from build123d import *

# Parameters (mm, degrees)
SKETCH1_W           = 152.4
SKETCH1_H           = 101.6
BOSS_EXTRUDE1_DEPTH = 6.35
SKETCH2_R           = 3.81
BOSS_EXTRUDE2_DEPTH = 50.8
SKETCH3_R           = 1.1303
CUT_EXTRUDE2_DEPTH  = 12.7
CUT_EXTRUDE3_DEPTH  = 6.35
SKETCH6_W           = 30.413113892
SKETCH6_H           = 50.8
BOSS_EXTRUDE3_DEPTH = 25.4
SKETCH8_W           = 30.413113892
SKETCH8_H           = 50.8
CUT_EXTRUDE4_DEPTH  = 25.4
SKETCH9_R           = 3.175
CUT_EXTRUDE5_DEPTH  = 2.54
SKETCH10_W          = 19.812
SKETCH10_H          = 64.262
CUT_EXTRUDE6_DEPTH  = 2.54
SKETCH12_R          = 1.1303
CUT_EXTRUDE7_DEPTH  = 132.950059198
FILLET1_R           = 2.54


with BuildPart() as part:
    # Sketch1 → Boss-Extrude1 (new body)
    with BuildSketch(Plane(origin=(0, 0, 0), x_dir=(1, 0, 0), z_dir=(0, 1, 0))):
        with Locations((28.027586207, -12.182445141)):
            Rectangle(SKETCH1_W, SKETCH1_H)
    extrude(amount=BOSS_EXTRUDE1_DEPTH)

    # Sketch2 → Boss-Extrude2 (add)
    with BuildSketch(Plane(origin=(0, 6.35, 0), x_dir=(1, 0, 0), z_dir=(0, 1, 0))):
        with Locations(Location((-44.362413793, 13.217554859, 0), (0, 0, 180))):
            Circle(SKETCH2_R)
        with Locations(Location((-43.092413793, -24.882445141, 0), (0, 0, 270))):
            Circle(SKETCH2_R)
        with Locations(Location((94.067586207, 19.567554859, 0), (0, 0, 270))):
            Circle(SKETCH2_R)
        with Locations(Location((94.067586207, -43.932445141, 0), (0, 0, 270))):
            Circle(SKETCH2_R)
    extrude(amount=BOSS_EXTRUDE2_DEPTH)

    # Sketch3 → Cut-Extrude2 (cut)
    with BuildSketch(Plane(origin=(0, 57.15, 0), x_dir=(1, 0, 0), z_dir=(0, 1, 0))):
        with Locations(Location((-44.362413793, 13.217554859, 0), (0, 0, 270))):
            Circle(SKETCH3_R)
        with Locations(Location((94.067586207, -43.932445141, 0), (0, 0, 270))):
            Circle(SKETCH3_R)
        with Locations(Location((94.067586207, 19.567554859, 0), (0, 0, 270))):
            Circle(SKETCH3_R)
        with Locations(Location((-43.092413793, -24.882445141, 0), (0, 0, 270))):
            Circle(SKETCH3_R)
    extrude(amount=-CUT_EXTRUDE2_DEPTH, mode=Mode.SUBTRACT)

    # Sketch4 → Cut-Extrude3 (cut)
    with BuildSketch(Plane.XZ):
        with BuildLine():
            ThreePointArc((38.123586207, 42.789445141), (37.537799769, 44.203658703), (36.123586207, 44.789445141))
            Line((36.123586207, 44.789445141), (36.123586207, 42.789445141))
            Line((36.123586207, 42.789445141), (36.123586207, 40.789445141))
            ThreePointArc((36.123586207, 40.789445141), (37.537799769, 41.375231579), (38.123586207, 42.789445141))
        make_face()
        with BuildLine():
            Line((36.123586207, 42.789445141), (36.123586207, 44.789445141))
            ThreePointArc((36.123586207, 44.789445141), (34.123586207, 42.789445141), (36.123586207, 40.789445141))
            Line((36.123586207, 40.789445141), (36.123586207, 42.789445141))
        make_face()
        with BuildLine():
            ThreePointArc((38.123586207, 42.789445141), (37.537799769, 44.203658703), (36.123586207, 44.789445141))
            Line((36.123586207, 44.789445141), (36.123586207, 42.789445141))
            Line((36.123586207, 42.789445141), (36.123586207, 40.789445141))
            ThreePointArc((36.123586207, 40.789445141), (37.537799769, 41.375231579), (38.123586207, 42.789445141))
        make_face()
        with BuildLine():
            Line((36.123586207, 42.789445141), (36.123586207, 44.789445141))
            ThreePointArc((36.123586207, 44.789445141), (34.123586207, 42.789445141), (36.123586207, 40.789445141))
            Line((36.123586207, 40.789445141), (36.123586207, 42.789445141))
        make_face()
        with BuildLine():
            ThreePointArc((45.426586207, 42.789445141), (44.840799769, 44.203658703), (43.426586207, 44.789445141))
            Line((43.426586207, 44.789445141), (43.426586207, 42.789445141))
            Line((43.426586207, 42.789445141), (43.426586207, 40.789445141))
            ThreePointArc((43.426586207, 40.789445141), (44.840799769, 41.375231579), (45.426586207, 42.789445141))
        make_face()
        with BuildLine():
            Line((43.426586207, 42.789445141), (43.426586207, 44.789445141))
            ThreePointArc((43.426586207, 44.789445141), (41.426586207, 42.789445141), (43.426586207, 40.789445141))
            Line((43.426586207, 40.789445141), (43.426586207, 42.789445141))
        make_face()
        with BuildLine():
            ThreePointArc((45.426586207, 42.789445141), (44.840799769, 44.203658703), (43.426586207, 44.789445141))
            Line((43.426586207, 44.789445141), (43.426586207, 42.789445141))
            Line((43.426586207, 42.789445141), (43.426586207, 40.789445141))
            ThreePointArc((43.426586207, 40.789445141), (44.840799769, 41.375231579), (45.426586207, 42.789445141))
        make_face()
        with BuildLine():
            Line((43.426586207, 42.789445141), (43.426586207, 44.789445141))
            ThreePointArc((43.426586207, 44.789445141), (41.426586207, 42.789445141), (43.426586207, 40.789445141))
            Line((43.426586207, 40.789445141), (43.426586207, 42.789445141))
        make_face()
    cut_extrude3 = extrude(amount=-CUT_EXTRUDE3_DEPTH, mode=Mode.SUBTRACT)

    # Sketch6 → Boss-Extrude3 (add)
    with BuildSketch(Plane(origin=(0, 6.35, 0), x_dir=(1, 0, 0), z_dir=(0, 1, 0))):
        with Locations((33.36893454, 13.217554859)):
            Rectangle(SKETCH6_W, SKETCH6_H)
    extrude(amount=BOSS_EXTRUDE3_DEPTH)

    # Mirror1: Cut-Extrude3 across plane
    add(cut_extrude3.mirror(Plane(origin=(48.575491486, 31.75, 12.182445141), x_dir=(1, 0, 0), z_dir=(0, 0, -1))), mode=Mode.SUBTRACT)

    # Sketch8 → Cut-Extrude4 (cut)
    with BuildSketch(Plane(origin=(0, 31.75, 0), x_dir=(1, 0, 0), z_dir=(0, 1, 0))):
        with Locations((33.36893454, 13.217554859)):
            Rectangle(SKETCH8_W, SKETCH8_H)
    extrude(amount=-CUT_EXTRUDE4_DEPTH, mode=Mode.SUBTRACT)

    # Sketch9 → Cut-Extrude5 (cut)
    with BuildSketch(Plane(origin=(0, 6.35, 0), x_dir=(1, 0, 0), z_dir=(0, 1, 0))):
        with Locations(Location((43.426586207, 18.424554859, 0), (0, 0, 270))):
            Circle(SKETCH9_R)
        with Locations(Location((36.123586207, 18.424554859, 0), (0, 0, 270))):
            Circle(SKETCH9_R)
        with Locations(Location((43.426586207, -42.789445141, 0), (0, 0, 270))):
            Circle(SKETCH9_R)
        with Locations(Location((36.123586207, -42.789445141, 0), (0, 0, 270))):
            Circle(SKETCH9_R)
    extrude(amount=-CUT_EXTRUDE5_DEPTH, mode=Mode.SUBTRACT)

    # Sketch10 → Cut-Extrude6 (cut)
    with BuildSketch(Plane(origin=(0, 6.35, 0), x_dir=(1, 0, 0), z_dir=(0, 1, 0))):
        with Locations((77.811586207, -9.756234071)):
            Rectangle(SKETCH10_W, SKETCH10_H)
    extrude(amount=-CUT_EXTRUDE6_DEPTH, mode=Mode.SUBTRACT)

    # Sketch12 → Cut-Extrude7 (cut, through all)
    with BuildSketch(Plane(origin=(0, 6.35, 0), x_dir=(1, 0, 0), z_dir=(0, 1, 0))):
        with Locations(Location((-31.662413793, 13.217554859, 0), (0, 0, 270))):
            Circle(SKETCH12_R)
        with Locations(Location((16.597586207, 11.947554859, 0), (0, 0, 270))):
            Circle(SKETCH12_R)
        with Locations(Location((1.357586207, -38.852445141, 0), (0, 0, 270))):
            Circle(SKETCH12_R)
        with Locations(Location((-26.582413793, -38.852445141, 0), (0, 0, 270))):
            Circle(SKETCH12_R)
    extrude(amount=-CUT_EXTRUDE7_DEPTH, mode=Mode.SUBTRACT)

    # Fillet1
    fillet1_edges = [part.edges().sort_by_distance(p)[0] for p in [
        (-48.172413793, 3.175, -38.617554859),
        (104.227586207, 3.175, -38.617554859),
        (104.227586207, 3.175, 62.982445141),
        (-48.172413793, 3.175, 62.982445141),
    ]]
    fillet(fillet1_edges, radius=FILLET1_R)


solid = part.part
CAD build for the part. Positions are in the model's coordinates, mm. A direction names the side the tool comes from. Coordinates: 2 decimals unless noted, no trailing zeros. Order: outer loops, then holes, each group sorted by start corner. A loop starts at its lowest first (then second) coordinate and runs counter-clockwise, first axis right, second up.
Item 1: Band-saw the part on A-A on z = 31. List the corners of the cut face in (x, y).
Check sheet entries:
outline: (-48.17, 0) - (104.23, 0) - (104.23, 6.35) - (87.72, 6.35) - (87.72, 3.81) - (67.91, 3.81) - (67.91, 6.35) - (-48.17, 6.35) - close
Item 2: 3-axis set-ups, long thin cutter, end or side, ignore diameter. For faces 4 (the face through (34.908, 5.098, 45.722)), 5 (the face through (-42, 57.15, 26)): which of +Z, -Z, +X, -X, +Y, -Y reach the whole face in a straight line?
Check sheet entries:
face 4: +Y
face 5: +Z, -Z, +X, -X, +Y
Item 3: Pin check, flat tips, straight feed: pin 1 Ø10 at (y, z) = (15.5, -26.5) entering from -X; pin 2 Ø3.5 at (x, z) = (-31.66, -13.22) entering from +Y; pin 3 Ø5.5 at (x, z) = (43.43, -18.42) entering from +Y. Stop position of each tip, or through.
Check sheet entries:
pin 1: stops at x = 90.78
pin 2: stops at y = 6.35
pin 3: stops at y = 3.81
Item 4: Band-saw the part on C-C on y = 14.5. List the corners of the cut face in (x, z), plus the area to 3 significant figures.
Check sheet entries:
outline: circle Ø7.62 at (-44.36, -13.22); circle Ø7.62 at (-43.09, 24.88); circle Ø7.62 at (94.07, -19.57); circle Ø7.62 at (94.07, 43.93)
area: 182 mm2
Item 5: Two-plate mould, pull along Z, no slides. Class faces 1 (the face through (36, 3.81, 45)), 2 (the face through (27, 3, -38.618)), 3 (the face through (93, 57.15, 43)): +Z half, -Z half, draft (parallel to the pull), parting line (faces both ways), or undercut.
Check sheet entries:
face 1: undercut
face 2: -Z half
face 3: draft
Item 6: Band-saw the part on D-D on x = -34.5. List the corners of the cut face in (y, z).
Check sheet entries:
outline: (0, -38.62) - (6.35, -38.62) - (6.35, 62.98) - (0, 62.98) - close
Item 7: Band-saw the part on B-B on x = 72. List the corners of the cut face in (y, z).
Check sheet entries:
outline: (0, -38.62) - (6.35, -38.62) - (6.35, -22.37) - (3.81, -22.37) - (3.81, 41.89) - (6.35, 41.89) - (6.35, 62.98) - (0, 62.98) - close
Item 8: Drill centre lines: L1, parallel to Y at x = -8.5, z = 41; L2, parallel to X at y = 47, z = 43.5; L3, parallel to X at y = 20, z = 25. Where is each one in solid material? Low to high.
Check sheet entries:
L1: y = 0 to 6.35
L2: x = 90.28 to 93.02, 95.11 to 97.85
L3: x = -46.9 to -39.28
